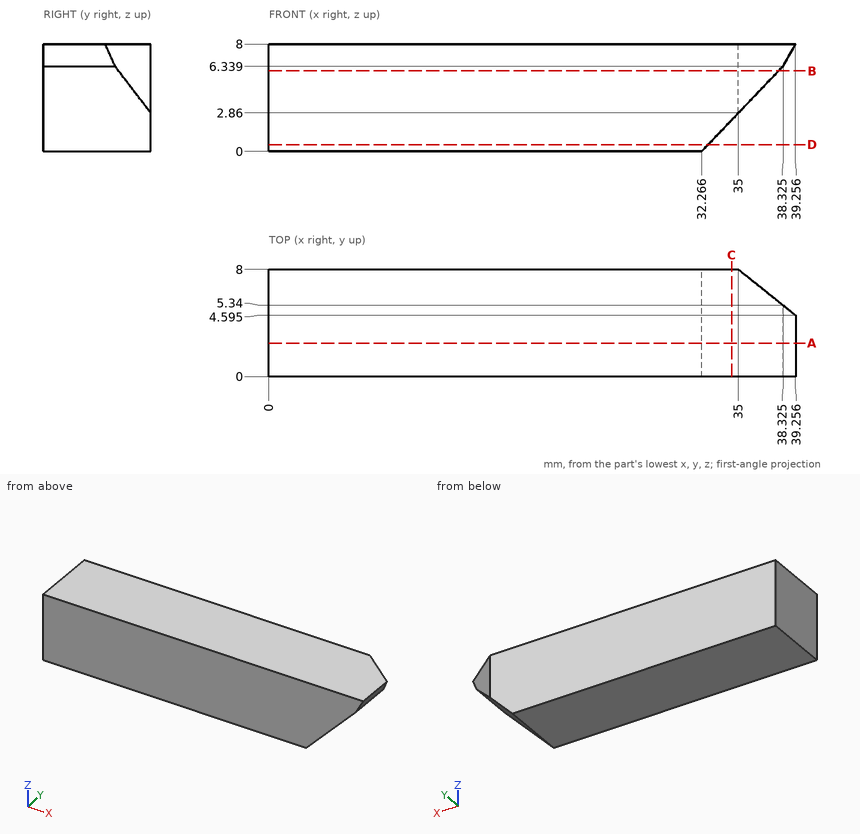
Drawing for the job (mm, zero at the part's lowest x, y, z). Coordinates: 2 decimals unless noted, no trailing zeros. Write each loop counter-clockwise with the first axis right and the second up, starting at its lowest first coordinate (ties: lowest second). Pieces come first, ordered by that corner, then holes. Notation, with made-up numbers: (74, -11.5) -> (108, -11.5) arc R37 ccw to (108, 24.5) -> close; hole circle Ø6 at (10, -18.5). An arc over 180 degrees is marked (long way). One line per item, written item: value. Start each with the question number.
1) Probe probe 1 along X at (y, z) = (7.75, 5.5) (1 decimal); probe 2 along Z at (x, y) = (35.5, 5) (1 decimal); probe 3 along X at (y, z) = (1.25, 2.75) (1 decimal). List the from-to ranges inside material, lowest first.
2) Slice it at A-A on y = 2.5. Write the cut outline in (x, z) (1 decimal), then the cut area to 3 significant figures.
3) Slice it at C-C on x = 34.5. Write the cut outline in (y, z).
4) Slice it at D-D on z = 0.5. Write the cut outline in (x, y), then the cut area to 3 significant figures.
5) Slice it at B-B on z = 6. Write the cut outline in (x, y).
6) Flat gauge pin, fed straight in: pin 1 Ø1 at (y, z) = (6, 4.5) entering from +X (1 decimal). Where does the tip first touch, or does it go through?
Answers follow:
1. probe 1: 0 to 35.3
1. probe 2: 3.4 to 8
1. probe 3: 0 to 34.9
2. outline: (0, 0) -> (32.3, 0) -> (38.3, 6.3) -> (39.3, 8) -> (0, 8) -> close
2. area: 288 mm2
3. outline: (0, 2.34) -> (8, 2.34) -> (8, 8) -> (0, 8) -> close
4. outline: (0, 0) -> (32.74, 0) -> (32.74, 8) -> (0, 8) -> close
4. area: 262 mm2
5. outline: (0, 0) -> (38, 0) -> (38, 5.6) -> (35, 8) -> (0, 8) -> close
6. pin 1: x = 37
